Source: CAD feature listing. Evaluate the final solid. Frame: model axes, mm. Face numbers are marked on the shaded views. A direction names the side the tool comes from. Round coordinates to 2 decimals unless told otherwise and drop trailing zeros. Order: outer loops, then holes, each group sorted by start corner. A loop starts at its lowest first (then second) coordinate and runs counter-clockwise, first axis right, second up. Notation, with made-up numbers: M 77,82.25 L 82,82.25 A15 ccw 82,109.25 Z; hole C -14.5,54 d9. An arc over 180 degrees is marked long. Answer as CSV lines item,"result". Start each with the question number.
Item 1: First-contact query: P1, Ø1, axis at x = -46, y = -46, coming from the -Z side; P2, Ø12, axis at x = -17, y = -47.5, coming from the -Z side; P3, Ø8, axis at x = 31.5, y = 23.5, coming from the -Z side. Flat tips, straight axial feed; report the tip coordinate or a pass-through.
Item 2: Set-up query: the marked faces 4, 5 and 6. Return all of +Z, -Z, +X, -X, +Y, -Y with unobstructed straight access to the full face (end or side cutting, diameter ignored); none if empty.
Item 3: Section query B-B on z = 9. Return the cut outline in (x, y).
Item 4: Pull-direction query (X, two-part tool) for the marked faces 1, 2 and 3; classes: +X half, -X half, draft (parallel to the pull), parting line (faces both ways), or undercut.
Item 5: Line query: line 1 (X direction, y = 19, z = 44.5); line 2 (Y direction, x = 45.5, z = 23.5); line 3 (Y direction, x = 26, z = 46). Output: solid intervals per line, ascending. Write a range as [from, to].
Item 6: Section query C-C on y = 35. Return the cut outline in (x, z).
Item 7: Section query A-A on x = -56. Return the cut outline in (y, z).
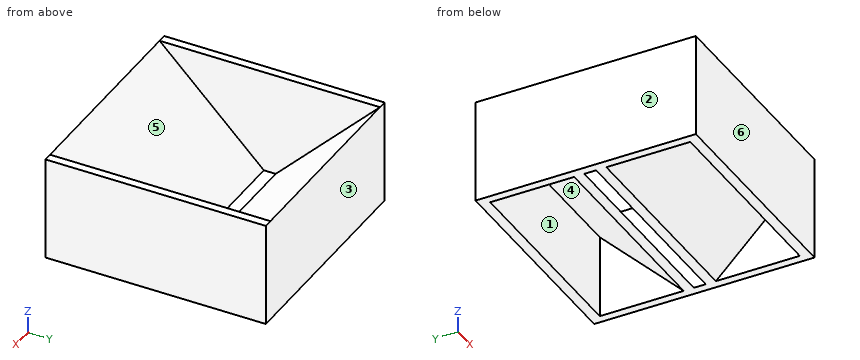
from build123d import *

# Parameters (mm, degrees)
BOSS_EXTRUDE1_DEPTH        = 60
BOSS_EXTRUDE1_DEPTH_BACK   = 60
BOSS_EXTRUDE1_2_DEPTH      = 60
BOSS_EXTRUDE1_2_DEPTH_BACK = 60
SKETCH2_W                  = 130
SKETCH2_H                  = 61.5
BOSS_EXTRUDE2_DEPTH        = 5


with BuildPart() as part:
    # Sketch1 → Boss-Extrude1 (new, two sides: drawn at the far end of the back side and taken through both)
    with BuildSketch(Plane.YZ.offset(-BOSS_EXTRUDE1_DEPTH_BACK)):
        Polygon((3.5, 0), (65, 61.5), (65, 0), (59, 0), (59, 49.5), (9.5, 0), align=None)
    extrude(amount=BOSS_EXTRUDE1_DEPTH + BOSS_EXTRUDE1_DEPTH_BACK)



with BuildPart() as body_2:
    # Sketch1 → Boss-Extrude1 2 (new, two sides: drawn at the far end of the back side and taken through both)
    with BuildSketch(Plane.YZ.offset(-BOSS_EXTRUDE1_2_DEPTH_BACK)):
        Polygon((-65, 61.5), (-3.5, 0), (-9.5, 0), (-59, 49.5), (-59, 0), (-65, 0), align=None)
    extrude(amount=BOSS_EXTRUDE1_2_DEPTH + BOSS_EXTRUDE1_2_DEPTH_BACK)


with BuildPart() as part_1:
    add(part.part)

    add(body_2.part)  # Boss-Extrude2 merges body 2
    # Sketch2 → Boss-Extrude2 (add)
    with BuildSketch(Plane.YZ.offset(60)):
        with Locations((0, 30.75)):
            Rectangle(SKETCH2_W, SKETCH2_H)
    boss_extrude2 = extrude(amount=BOSS_EXTRUDE2_DEPTH)

    # Mirror1: Boss-Extrude2 across plane
    add(boss_extrude2.mirror(Plane(origin=(0, 0, 0), x_dir=(0, 0, 1), z_dir=(1, 0, 0))))


solid = part_1.part
Results:
1,P1,"z = 36"
1,P2,"z = 32"
1,P3,"z = 10"
2,face 4,"-Z"
2,face 5,"+Z"
2,face 6,"+Z, -Z, +X, -X, -Y"
3,outline,"M -65,-65 L 65,-65 L 65,65 L -65,65 Z; hole M -60,-59 L 60,-59 L 60,-18.5 L -60,-18.5 Z; hole M -60,-12.5 L 60,-12.5 L 60,12.5 L -60,12.5 Z; hole M -60,18.5 L 60,18.5 L 60,59 L -60,59 Z"
4,face 1,"undercut"
4,face 2,"-X half"
4,face 3,"draft"
5,line 1,"[-65, -60], [60, 65]"
5,line 2,"[-65, -59], [-33, -27], [27, 33], [59, 65]"
5,line 3,"[-65, -59], [-55.5, -49.5], [49.5, 55.5], [59, 65]"
6,outline,"M -65,0 L -60,0 L -60,25.5 L 60,25.5 L 60,0 L 65,0 L 65,61.5 L 60,61.5 L 60,31.5 L -60,31.5 L -60,61.5 L -65,61.5 Z"
7,outline,"M -65,0 L -59,0 L -59,49.5 L -9.5,0 L -3.5,0 L -65,61.5 Z; M 3.5,0 L 9.5,0 L 59,49.5 L 59,0 L 65,0 L 65,61.5 Z"
